For this review, take the finished solid that the model builds, in its own axes (mm). Coordinates: 2 decimals unless noted, no trailing zeros. Order: outer loops, then holes, each group sorted by start corner. A loop starts at its lowest first (then second) coordinate and runs counter-clockwise, first axis right, second up.
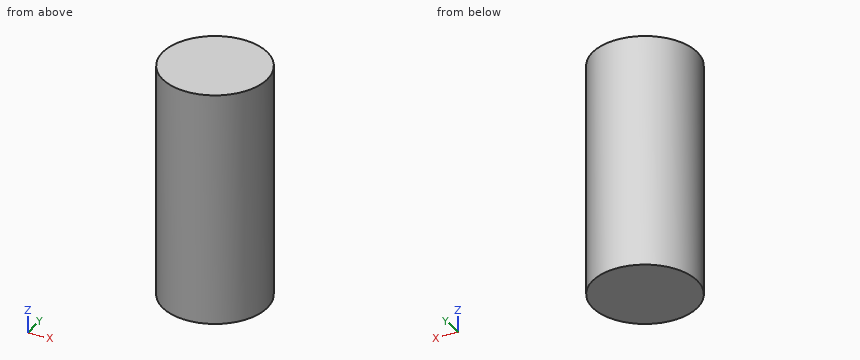
from build123d import *

# Parameters (mm, degrees)
SCHIZZO1_R                   = 58.7
ESTRUSIONE_ESTRUSIONE1_DEPTH = 5
SCHIZZO2_R                   = 58.7
SCHIZZO2_R_2                 = 48.7
ESTRUSIONE_ESTRUSIONE2_DEPTH = 254
SCHIZZO3_R                   = 58.7
ESTRUSIONE_ESTRUSIONE3_DEPTH = 5


with BuildPart() as part:
    # Schizzo1 → Estrusione-Estrusione1 (new body)
    with BuildSketch(Plane.XY):
        Circle(SCHIZZO1_R)
    extrude(amount=ESTRUSIONE_ESTRUSIONE1_DEPTH)

    # Schizzo2 → Estrusione-Estrusione2 (add)
    with BuildSketch(Plane.XY.offset(5)):
        Circle(SCHIZZO2_R)
        Circle(SCHIZZO2_R_2, mode=Mode.SUBTRACT)
    extrude(amount=ESTRUSIONE_ESTRUSIONE2_DEPTH)

    # Schizzo3 → Estrusione-Estrusione3 (add)
    with BuildSketch(Plane.XY.offset(259)):
        Circle(SCHIZZO3_R)
    extrude(amount=ESTRUSIONE_ESTRUSIONE3_DEPTH)


solid = part.part
1. Take a section at C-C, the plane z = 65. Give the boundary of the cut face in (x, y), plus the area to 3 significant figures.
Answer below:
outline: circle Ø117.4 at (0, 0); hole circle Ø97.4 at (0, 0)
area: 3,370 mm2
2. To check wall thickness, follow L1, parallel to Z at x = 3.5, y = -32; L2, parallel to Y at x = 0, z = 206; L3, parallel to Y at x = -30, z = 118.5. State the ranges of each line that lie inside material, in increasing order.
Answer below:
L1: z = 0 to 5, 259 to 264
L2: y = -58.7 to -48.7, 48.7 to 58.7
L3: y = -50.45 to -38.36, 38.36 to 50.45
3. Take a section at A-A, the plane x = 0. Give the boundary of the cut face in (y, z), plus the area to 3 significant figures.
Answer below:
outline: (-58.7, 0) - (58.7, 0) - (58.7, 264) - (-58.7, 264) - close; hole (-48.7, 5) - (48.7, 5) - (48.7, 259) - (-48.7, 259) - close
area: 6,250 mm2
4. Clearance check with flat-ended pins moving along their axes: pin 1 Ø1 at (y, z) = (39.5, 187) entering from -X; pin 2 Ø5 at (x, z) = (17, 70) entering from -Y; pin 3 Ø1.5 at (x, z) = (27, 143) entering from +Y. State where each tip first meets the part, or that it passes through.
Answer below:
pin 1: stops at x = -43.87
pin 2: stops at y = -56.88
pin 3: stops at y = 52.5
